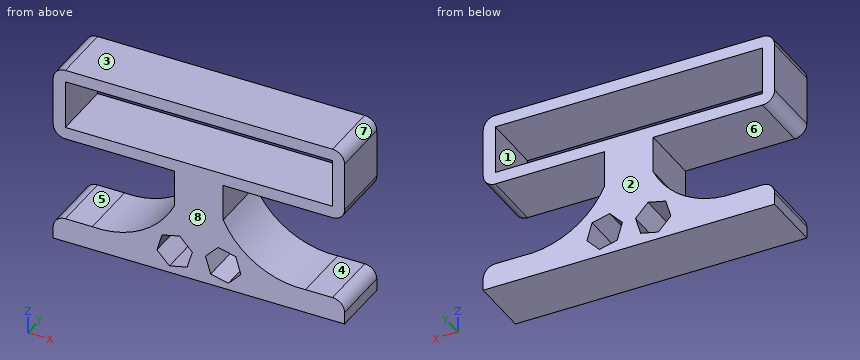
from build123d import *

# Parameters (mm, degrees)
F1_DEPTH = 25


with BuildPart() as f1:
    # F0 (on Front) → F1 (new body)
    with BuildSketch(Plane.XZ):
        with BuildLine():
            Line((-60, 0), (0, 0))
            Line((0, 0), (60, 0))
            Line((60, 0), (60, 5))
            ThreePointArc((60, 5), (58.535534, 8.535534), (55, 10))
            Line((55, 10), (43.900207, 10))
            ThreePointArc((43.900207, 10), (23.870935, 14.706872), (10, 29.903039))
            Line((10, 29.903039), (10, 45))
            Line((10, 45), (55, 45))
            ThreePointArc((55, 45), (58.535534, 46.464466), (60, 50))
            Line((60, 50), (60, 70))
            ThreePointArc((60, 70), (58.535534, 73.535534), (55, 75))
            Line((55, 75), (0, 75))
            Line((0, 75), (-55, 75))
            ThreePointArc((-55, 75), (-58.535534, 73.535534), (-60, 70))
            Line((-60, 70), (-60, 50))
            ThreePointArc((-60, 50), (-58.535534, 46.464466), (-55, 45))
            Line((-55, 45), (-10, 45))
            Line((-10, 45), (-10, 29.903039))
            ThreePointArc((-10, 29.903039), (-23.870935, 14.706872), (-43.900207, 10))
            Line((-43.900207, 10), (-55, 10))
            ThreePointArc((-55, 10), (-58.535534, 8.535534), (-60, 5))
            Line((-60, 5), (-60, 0))
        make_face()
        Polygon((-12.136564, 2.810765), (-17.294342, 8.255701), (-15.157778, 15.444936), (-7.863436, 17.189235), (-2.705658, 11.744299), (-4.842222, 4.555064), align=None, mode=Mode.SUBTRACT)
        Polygon((15.157778, 15.444936), (17.294342, 8.255701), (12.136564, 2.810765), (4.842222, 4.555064), (2.705658, 11.744299), (7.863436, 17.189235), align=None, mode=Mode.SUBTRACT)
        Polygon((-55, 70), (0, 70), (55, 70), (55, 50), (0, 50), (-55, 50), align=None, mode=Mode.SUBTRACT)
    extrude(amount=F1_DEPTH)


solid = f1.part
Input: part model. Units: mm. Frame: model coordinates. Face numbers are marked on the shaded views. A direction names the side the tool comes from. Round coordinates to 2 decimals unless told otherwise and drop trailing zeros. Loops run counter-clockwise (first coordinate to the right, second up) from the corner with the lowest first, then second, coordinate; pieces in that order, holes last. Notation, with made-up numbers: M 20.25,40.5 L 61.25,40.5 A21 ccw 61.25,72.5 Z; hole C 74,-28.75 d10. An arc over 180 degrees is marked long. Answer as CSV lines item,"result". Start each with the question number.
(1) Section A-A, the plane z = 67.5. Output: boundary loops of the cut face in (x, y).
(2) Section D-D, the plane y = -11. State how many separate pieces and enclosed holes the cut face has, plus the area to 3 significant figures.
(3) Line query: line 1 (Z direction, x = -49, y = -3.75); line 2 (X direction, y = -8, z = 69.5); line 3 (Z direction, x = 18.5, y = -19.5). Output: solid intervals per line, ascending. Write a range as [from, to].
(4) Section C-C, the plane x = 20. Output: boundary loops of the cut face in (y, z).
(5) Reachability of the marked faces 1, 2, 3, 4 and 5 from +Z, -Z, +X, -X, +Y, -Y: full face, straight path, thin tool, end or side. Return the list, or none.
(6) Draft query along Z for the marked faces 6, 7 and 8. Return one class per face: released by +Z, released by -Z, zero draft, split by the parting line, or undercut.
(7) Section B-B, the plane x = -51. Output: boundary loops of the cut face in (y, z).
(8) First-contact query: pin 1 (6 mm diameter, centred on y = -13, z = 39, fed in from +X); pin 2 (6 mm diameter, centred on y = -18, z = 17, fed in from +X); pin 3 (12 mm diameter, centred on y = -13, z = 39.5, fed in from +X). Flat tips, straight axial feed; report the tip coordinate or a pass-through.
Values found:
1,outline,"M -60,-25 L -55,-25 L -55,0 L -60,0 Z; M 55,-25 L 60,-25 L 60,0 L 55,0 Z"
2,separate pieces,"1"
2,enclosed holes,"3"
2,area,"3,330 mm²"
3,line 1,"z = [0, 10], [45, 50], [70, 75]"
3,line 2,"x = [-60, -55], [55, 60]"
3,line 3,"z = [0, 18.59], [45, 50], [70, 75]"
4,outline,"M -25,0 L 0,0 L 0,17.35 L -25,17.35 Z; M -25,45 L 0,45 L 0,50 L -25,50 Z; M -25,70 L 0,70 L 0,75 L -25,75 Z"
5,face 1,"+Y, -Y"
5,face 2,"+Z, -Z, +X, -X, +Y"
5,face 3,"+Z, +X, -X, +Y, -Y"
5,face 4,"+X, +Y, -Y"
5,face 5,"-X, +Y, -Y"
6,face 6,"undercut"
6,face 7,"released by +Z"
6,face 8,"zero draft"
7,outline,"M -25,0 L 0,0 L 0,10 L -25,10 Z; M -25,45 L 0,45 L 0,50 L -25,50 Z; M -25,70 L 0,70 L 0,75 L -25,75 Z"
8,pin 1,"stops at x = 10"
8,pin 2,"stops at x = 25.13"
8,pin 3,"stops at x = 57.18"
